```python
from build123d import *

# Parameters (mm, degrees)
SKETCH1_W           = 60
SKETCH1_H           = 43
SKETCH1_R           = 1.65
BOSS_EXTRUDE1_DEPTH = 3
CUT_EXTRUDE1_DEPTH  = 38.030392923


with BuildPart() as part:
    # Sketch1 → Boss-Extrude1 (new body)
    with BuildSketch(Plane.XY):
        Rectangle(SKETCH1_W, SKETCH1_H)
        with Locations((-25, 17.5)):
            Circle(SKETCH1_R, mode=Mode.SUBTRACT)
        with Locations((25, 17.5)):
            Circle(SKETCH1_R, mode=Mode.SUBTRACT)
        with Locations((25, -17.5)):
            Circle(SKETCH1_R, mode=Mode.SUBTRACT)
        with Locations((-25, -17.5)):
            Circle(SKETCH1_R, mode=Mode.SUBTRACT)
    extrude(amount=BOSS_EXTRUDE1_DEPTH)

    # Sketch2 → Cut-Extrude1 (cut, through all)
    with BuildSketch(Plane(origin=(0, 0, 0), x_dir=(-1, 0, 0), z_dir=(0, 0, -1))):
        with BuildLine():
            Line((15, -2.75), (5, -2.75))
            ThreePointArc((5, -2.75), (2.25, 0), (5, 2.75))
            Line((5, 2.75), (15, 2.75))
            ThreePointArc((15, 2.75), (17.75, 0), (15, -2.75))
        make_face()
    extrude(amount=-CUT_EXTRUDE1_DEPTH, mode=Mode.SUBTRACT)


solid = part.part
```
Geometry check sheet. Reference: the model listing, model coordinates, mm. A direction names the side the tool comes from. Give positions to 0.01 mm unless a question says otherwise; leave off trailing zeros. Write each loop counter-clockwise with the first axis right and the second up, starting at its lowest first coordinate (ties: lowest second). Pieces come first, ordered by that corner, then holes.
1) Section check C-C, the plane x = -25. Record the boundary of the cut face in (y, z), and give its area (3 significant figures).
2) Section check D-D, the plane y = 0. Record the boundary of the cut face in (x, z), and give its area (4 significant figures).
3) Access from +Z, -Z, +X, -X, +Y, -Y to the whole of each face (thin tool, end or side, straight path). Record for faces 4 (the flat face through (30, 0, 1)), 5 (the flat face through (-10, -2.75, 1)).
4) Gauge pin test, flat end, axial feed: pin 1 (3 mm diameter, centred on x = -25, y = -17.5, fed in from +Z). Record the tip position at first contact, or that the pin passes through.
5) Release check for a two-part mould opening along Y. For faces 1 (the flat face through (-30, 0, 1)), 2 (the cylindrical face through (-2.25, -0.06, 1.48)), 3 (the flat face through (0, 21.5, 1)) record: pulls with the +Y half, pulls with the -Y half, needs draft (parallel to the pull), parting line crosses it, or undercut.
6) Section check A-A, the plane y = -17.5. Record the boundary of the cut face in (x, z), and give its area (3 significant figures).
7) Material ranges on L1, parallel to Y at x = -25, z = 0.8; L2, parallel to Y at x = -26.5, z = 2.5; L3, parallel to Y at x = -4, z = 1.05, recorded low to high.
8) Section check B-B, the plane z = 0.75. Record the boundary of the cut face in (x, y), and give its area (3 significant figures).
Computed:
1. outline: (-21.5, 0) - (-19.15, 0) - (-19.15, 3) - (-21.5, 3) - close; (-15.85, 0) - (15.85, 0) - (15.85, 3) - (-15.85, 3) - close; (19.15, 0) - (21.5, 0) - (21.5, 3) - (19.15, 3) - close
1. area: 109 mm2
2. outline: (-30, 0) - (-17.75, 0) - (-17.75, 3) - (-30, 3) - close; (-2.25, 0) - (30, 0) - (30, 3) - (-2.25, 3) - close
2. area: 133.5 mm2
3. face 4: +Z, -Z, +X, +Y, -Y
3. face 5: +Z, -Z
4. pin 1: passes through
5. face 1: needs draft
5. face 2: undercut
5. face 3: pulls with the +Y half
6. outline: (-30, 0) - (-26.65, 0) - (-26.65, 3) - (-30, 3) - close; (-23.35, 0) - (23.35, 0) - (23.35, 3) - (-23.35, 3) - close; (26.65, 0) - (30, 0) - (30, 3) - (26.65, 3) - close
6. area: 160 mm2
7. L1: y = -21.5 to -19.15, -15.85 to 15.85, 19.15 to 21.5
7. L2: y = -21.5 to -18.19, -16.81 to 16.81, 18.19 to 21.5
7. L3: y = -21.5 to -2.56, 2.56 to 21.5
8. outline: (-30, -21.5) - (30, -21.5) - (30, 21.5) - (-30, 21.5) - close; hole circle Ø3.3 at (-25, -17.5); hole circle Ø3.3 at (-25, 17.5); hole (-15, -2.75) - (-5, -2.75) arc R2.75 ccw to (-5, 2.75) - (-15, 2.75) arc R2.75 ccw to start; hole circle Ø3.3 at (25, -17.5); hole circle Ø3.3 at (25, 17.5)
8. area: 2,470 mm2
